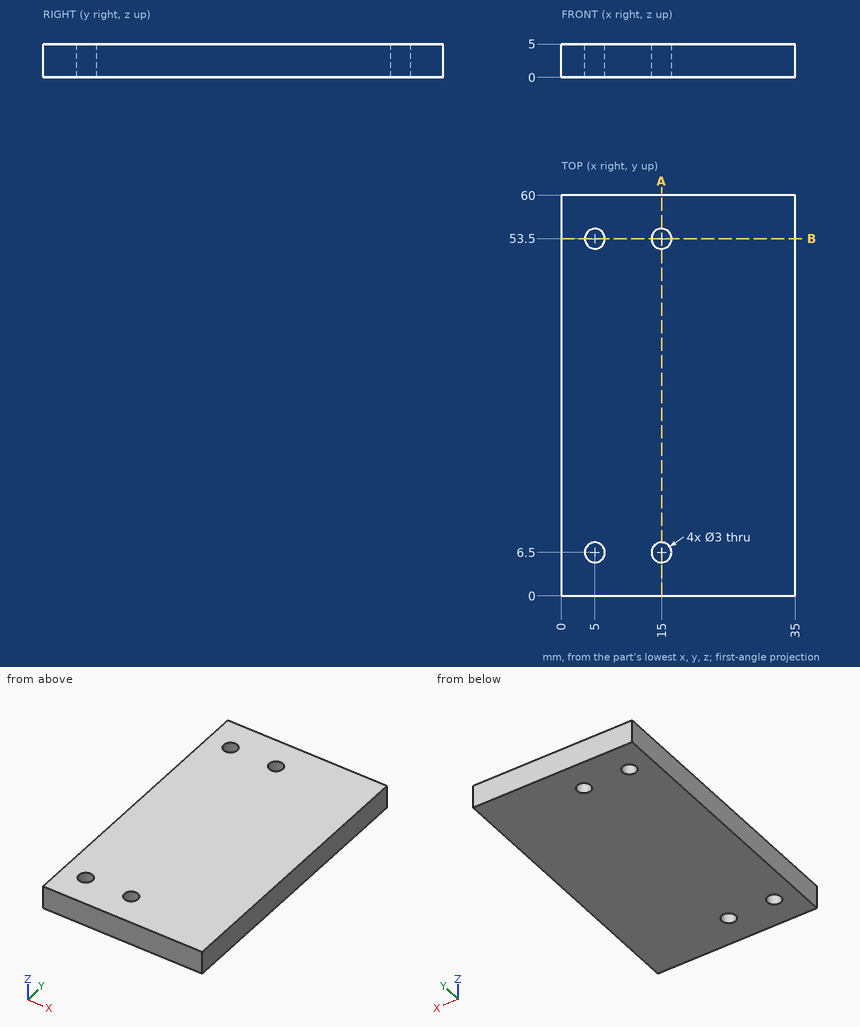
The figure shows three views and two pictorial views of one solid part (mm, origin at its lowest corner). Answer the questions. Round coordinates to 2 decimals unless told otherwise and drop trailing zeros. Order: outer loops, then holes, each group sorted by start corner. A loop starts at its lowest first (then second) coordinate and runs counter-clockwise, first axis right, second up.
Q1. A cutting plane is placed at B-B, the plane y = 53.5. Determine the outline of the cut face in (x, z), then the cut area to 3 significant figures.
Solution:
outline: (0, 0) - (3.5, 0) - (3.5, 5) - (0, 5) - close; (6.5, 0) - (13.5, 0) - (13.5, 5) - (6.5, 5) - close; (16.5, 0) - (35, 0) - (35, 5) - (16.5, 5) - close
area: 145 mm2
Q2. A cutting plane is placed at A-A, the plane x = 15. Determine the outline of the cut face in (y, z).
Solution:
outline: (0, 0) - (5, 0) - (5, 5) - (0, 5) - close; (8, 0) - (52, 0) - (52, 5) - (8, 5) - close; (55, 0) - (60, 0) - (60, 5) - (55, 5) - close
Q3. Given pin 1 Ø2.5 at (x, y) = (5, 53.5) entering from -Z, flat-ended and moving along its own axis, determine where the tip first touches the part or whether it passes through.
Solution:
pin 1: passes through
Q4. Find the intervals of material crossed by line 1 along Y through (x, z) = (5, 3.1); line 2 along Y through (x, z) = (4, 3.45), in increasing order.
Solution:
line 1: y = 0 to 5, 8 to 52, 55 to 60
line 2: y = 0 to 5.38, 7.62 to 52.38, 54.62 to 60
